Can you work these out from the model? Positions are in its coordinate system, mm. A direction names the side the tool comes from. Give positions to 0.01 mm unless a question says otherwise; leave off trailing zeros. Write each loop counter-clockwise with the first axis right and the second up, starting at its lowest first coordinate (ties: lowest second). Pieces come first, ordered by that corner, then holes. Notation, with made-up numbers: (8.25, 35) -> (63.25, 35) arc R20 cw to (63.25, 56) -> close; hole circle Ø1 at (70.5, 55.25). An arc over 180 degrees is marked (long way). One line per item, written item: value.
from build123d import *

# Parameters (mm, degrees)
SKETCH1_W             = 7.497163216
SKETCH1_H             = 13.3
SKETCH1_R             = 1
BOSS_EXTRUDE1_DEPTH   = 2
BOSS_EXTRUDE1_2_DEPTH = 2
SKETCH3_R             = 2.5
CUT_EXTRUDE1_DEPTH    = 1
BOSS_EXTRUDE3_DEPTH   = 1
SKETCH5_R             = 3.1
BOSS_EXTRUDE4_DEPTH   = 15.323280282
CUT_EXTRUDE2_REACH    = 37.51
SKETCH6_W             = 9.3
SKETCH6_H             = 13.397572085
BOSS_EXTRUDE5_START   = -13.397572085
BOSS_EXTRUDE5_DEPTH   = 13.397572085
SKETCH8_W             = 13.005673568
SKETCH8_H             = 3
BOSS_EXTRUDE6_DEPTH   = 10.5515
SKETCH9_W             = 13.3
SKETCH9_H             = 12.323280282
BOSS_EXTRUDE7_DEPTH   = 4
SKETCH10_W            = 4
SKETCH10_H            = 13.3
BOSS_EXTRUDE8_DEPTH   = 70
BOSS_EXTRUDE9_DEPTH   = 13.3
SKETCH15_W            = 4
SKETCH15_H            = 20
BOSS_EXTRUDE13_DEPTH  = 20
SKETCH16_W            = 4
SKETCH16_H            = 20
BOSS_EXTRUDE14_DEPTH  = 30
CUT_EXTRUDE3_DEPTH    = 20
BOSS_EXTRUDE15_DEPTH  = 4
BOSS_EXTRUDE16_DEPTH  = 20
SKETCH21_W            = 7.497163216
SKETCH21_H            = 9.3
CUT_EXTRUDE4_DEPTH    = 2
BOSS_EXTRUDE18_DEPTH  = 4
CUT_EXTRUDE5_DEPTH    = 4
BOSS_EXTRUDE20_DEPTH  = 8.1
FILLET1_R             = 5


with BuildPart() as part:
    # Sketch1 → Boss-Extrude1 (new body)
    with BuildSketch(Plane(origin=(0, 0, 0), x_dir=(1, 0, 0), z_dir=(0, 1, 0))):
        with Locations((6.360378056, -6.65)):
            Rectangle(SKETCH1_W, SKETCH1_H)
        with Locations(Location((6.360378056, -6.65, 0), (0, 0, 270))):
            Circle(SKETCH1_R, mode=Mode.SUBTRACT)
    extrude(amount=BOSS_EXTRUDE1_DEPTH)


with BuildPart() as body_2:
    # Sketch1 → Boss-Extrude1 2 (new body)
    with BuildSketch(Plane(origin=(0, 0, 0), x_dir=(1, 0, 0), z_dir=(0, 1, 0))):
        with Locations((26.86321484, -6.65)):
            Rectangle(SKETCH1_W, SKETCH1_H)
        with Locations(Location((26.86321484, -6.65, 0), (0, 0, 270))):
            Circle(SKETCH1_R, mode=Mode.SUBTRACT)
    extrude(amount=BOSS_EXTRUDE1_2_DEPTH)


with BuildPart() as cut_extrude1_tool:
    # Sketch3 → Cut-Extrude1 (new body)
    with BuildSketch(Plane(origin=(0, 2, 0), x_dir=(1, 0, 0), z_dir=(0, 1, 0))):
        with Locations(Location((26.86321484, -6.65, 0), (0, 0, 270))):
            Circle(SKETCH3_R)
        with Locations(Location((6.360378056, -6.65, 0), (0, 0, 270))):
            Circle(SKETCH3_R)
    extrude(amount=-CUT_EXTRUDE1_DEPTH)


with BuildPart() as part_1:
    add(part.part)

    # Cut-Extrude1: cut by cut_extrude1_tool
    add(cut_extrude1_tool.part, mode=Mode.SUBTRACT)



with BuildPart() as body_2_1:
    add(body_2.part)

    # Cut-Extrude1: cut by cut_extrude1_tool
    add(cut_extrude1_tool.part, mode=Mode.SUBTRACT)


with BuildPart() as part_2:
    add(part_1.part)

    add(body_2_1.part)  # Boss-Extrude3 merges body 2
    # Sketch4 → Boss-Extrude3 (add)
    with BuildSketch(Plane.XY.offset(13.3)):
        Polygon((10.108959664, 0), (10.108959664, -6.625791341), (23.114633232, -6.625791341), (23.114633232, 2), (10.108959664, 2), align=None)
    extrude(amount=-BOSS_EXTRUDE3_DEPTH)

    # Sketch5 → Boss-Extrude4 (add)
    with BuildSketch(Plane(origin=(0, 2, 0), x_dir=(1, 0, 0), z_dir=(0, 1, 0))):
        Polygon((10.108959664, 0), (2.611796448, 0), (2.611796448, -4), (2.611796448, -9.3), (2.611796448, -12.3), (2.611796448, -13.3), (30.611796448, -13.3), (30.611796448, -12.3), (30.611796448, -9.3), (30.611796448, -4), (30.611796448, 0), (23.114633232, 0), (23.114633232, -4), (23.114633232, -9.3), (23.114633232, -12.3), (10.108959664, -12.3), (10.108959664, -9.3), (10.108959664, -4), align=None)
        with Locations(Location((6.360378056, -6.65, 0), (0, 0, 270))):
            Circle(SKETCH5_R, mode=Mode.SUBTRACT)
        with Locations(Location((26.86321484, -6.65, 0), (0, 0, 270))):
            Circle(SKETCH5_R, mode=Mode.SUBTRACT)
    extrude(amount=BOSS_EXTRUDE4_DEPTH)

    # Cut-Extrude2: up to this face of the body (flat: up to its plane)
    cut_extrude2_end = Plane(part_2.part.faces().sort_by_distance((23.114633232, 8.661640141, 6.15))[0])
    # Sketch6 → Cut-Extrude2 (cut, up to the picked face)
    with BuildSketch(Plane(origin=(30.611796448, 0, 0), x_dir=(0, 0, -1), z_dir=(1, 0, 0)), mode=Mode.PRIVATE) as cut_extrude2_sk1:
        with Locations((-4.65, 10.62449424)):
            Rectangle(SKETCH6_W, SKETCH6_H)
    cut_extrude2_tool1 = split(extrude(cut_extrude2_sk1.sketch, amount=-CUT_EXTRUDE2_REACH, mode=Mode.PRIVATE), bisect_by=cut_extrude2_end, keep=Keep.BOTH, mode=Mode.PRIVATE)
    add(cut_extrude2_tool1.solids().sort_by(Axis((30.611796, 10.624494, 4.65), (-1, 0, 0)))[0], mode=Mode.SUBTRACT)

    # Sketch7 → Boss-Extrude5 (add)
    with BuildSketch(Plane(origin=(0, 17.323280282, 0), x_dir=(1, 0, 0), z_dir=(0, 1, 0)).offset(BOSS_EXTRUDE5_START)):
        with BuildLine():
            Line((28.471785634, -9.3), (30.611796448, -9.3))
            Line((30.611796448, -9.3), (30.611796448, -13.3))
            Line((30.611796448, -13.3), (10.108959664, -13.3))
            Line((10.108959664, -13.3), (10.108959664, -9.3))
            Line((10.108959664, -9.3), (25.254644046, -9.3))
            ThreePointArc((25.254644046, -9.3), (26.86321484, -9.75), (28.471785634, -9.3))
        make_face()
    extrude(amount=BOSS_EXTRUDE5_DEPTH)

    # Sketch8 → Boss-Extrude6 (add, through all)
    with BuildSketch(Plane.XZ.offset(-3.925708197)):
        with Locations((16.611796448, 10.8)):
            Rectangle(SKETCH8_W, SKETCH8_H)
    extrude(amount=BOSS_EXTRUDE6_DEPTH)

    # Sketch9 → Boss-Extrude7 (add)
    with BuildSketch(Plane.ZY.offset(-2.611796448)):
        with Locations((6.65, 11.161640141)):
            Rectangle(SKETCH9_W, SKETCH9_H)
    extrude(amount=BOSS_EXTRUDE7_DEPTH)

    # Sketch10 → Boss-Extrude8 (add)
    with BuildSketch(Plane(origin=(0, 17.323280282, 0), x_dir=(1, 0, 0), z_dir=(0, 1, 0))):
        with Locations((0.611796448, -6.65)):
            Rectangle(SKETCH10_W, SKETCH10_H)
    extrude(amount=BOSS_EXTRUDE8_DEPTH)

    # Sketch11 → Boss-Extrude9 (add)
    with BuildSketch(Plane.XY.offset(13.3)):
        Polygon((-1.388203552, 5), (2.611796448, 0), (2.611796448, 5), align=None)
    extrude(amount=-BOSS_EXTRUDE9_DEPTH)

    # Sketch15 → Boss-Extrude13 (add)
    with BuildSketch(Plane.XY.offset(13.3)):
        with Locations((0.611796448, 47.323280282)):
            Rectangle(SKETCH15_W, SKETCH15_H)
    extrude(amount=BOSS_EXTRUDE13_DEPTH)

    # Sketch16 → Boss-Extrude14 (add)
    with BuildSketch(Plane(origin=(0, 57.323280282, 0), x_dir=(1, 0, 0), z_dir=(0, 1, 0))):
        with Locations((0.611796448, -23.3)):
            Rectangle(SKETCH16_W, SKETCH16_H)
    extrude(amount=BOSS_EXTRUDE14_DEPTH)

    # Sketch17 → Cut-Extrude3 (cut)
    with BuildSketch(Plane.ZY.offset(1.388203552)):
        Polygon((13.3, 87.323280282), (0, 87.323280282), (0, 57.323280282), (0, 44.023280282), (13.3, 57.323280282), align=None)
        Polygon((33.3, 87.323280282), (26.6, 87.323280282), (26.6, 50.623280282), (13.3, 37.323280282), (26.6, 37.323280282), (33.3, 37.323280282), align=None)
    extrude(amount=-CUT_EXTRUDE3_DEPTH, mode=Mode.SUBTRACT)

    # Sketch18 → Boss-Extrude15 (add)
    with BuildSketch(Plane.ZY.offset(1.388203552)):
        Polygon((3.495517328, 77.823280282), (36.404482672, 96.823280282), (36.404482672, 92.823280282), (3.495517328, 73.823280282), align=None)
        Polygon((3.495517328, 56.502772207), (36.404482672, 75.502772207), (36.404482672, 71.502772207), (3.495517328, 52.502772207), align=None)
    extrude(amount=-BOSS_EXTRUDE15_DEPTH)

    # Sketch19 → Boss-Extrude16 (add)
    with BuildSketch(Plane.ZY.offset(1.388203552)):
        Polygon((3.495517328, 77.823280282), (6.959618943, 79.823280282), (6.959618943, 75.823280282), (3.495517328, 73.823280282), align=None)
        Polygon((3.495517328, 56.502772207), (6.959618943, 58.502772207), (6.959618943, 54.502772207), (3.495517328, 52.502772207), align=None)
        Polygon((36.404482672, 75.502772207), (32.940381057, 73.502772207), (32.940381057, 69.502772207), (36.404482672, 71.502772207), align=None)
        Polygon((36.404482672, 92.823280282), (32.940381057, 90.823280282), (32.940381057, 94.823280282), (36.404482672, 96.823280282), align=None)
    extrude(amount=BOSS_EXTRUDE16_DEPTH)

    # Sketch21 → Cut-Extrude4 (cut)
    with BuildSketch(Plane(origin=(0, 3.925708197, 0), x_dir=(1, 0, 0), z_dir=(0, 1, 0))):
        with Locations((26.86321484, -4.65)):
            Rectangle(SKETCH21_W, SKETCH21_H)
    extrude(amount=-CUT_EXTRUDE4_DEPTH, mode=Mode.SUBTRACT)

    # Sketch22 → Boss-Extrude18 (add)
    with BuildSketch(Plane.ZY.offset(21.388203552)):
        Polygon((3.495517328, 77.823280282), (36.404482672, 96.823280282), (36.404482672, 92.823280282), (3.495517328, 73.823280282), align=None)
        Polygon((3.495517328, 56.502772207), (3.495517328, 52.502772207), (36.404482672, 71.502772207), (36.404482672, 75.502772207), align=None)
    extrude(amount=BOSS_EXTRUDE18_DEPTH)

    # Sketch23 → Cut-Extrude5 (cut)
    with BuildSketch(Plane(origin=(2.611796448, 0, 0), x_dir=(0, 0, -1), z_dir=(1, 0, 0))):
        Polygon((-13.3, 87.323280282), (-13.3, 83.483900992), (-19.95, 87.323280282), align=None)
    extrude(amount=-CUT_EXTRUDE5_DEPTH, mode=Mode.SUBTRACT)

    # Sketch24 → Boss-Extrude20 (add)
    with BuildSketch(Plane(origin=(2.611796448, 0, 0), x_dir=(0, 0, -1), z_dir=(1, 0, 0))):
        Polygon((-26.6, 91.162659572), (-13.300321898, 83.48408684), (-13.3, 62.163392916), (-26.599678102, 69.841965649), align=None)
    extrude(amount=BOSS_EXTRUDE20_DEPTH)

    # Fillet1
    # the kernel refuses this fillet: 5 mm, written as the material it takes off along each edge
    with BuildSketch(Plane(origin=(30.611796448, 17.323280282, -3.2), x_dir=(-1, 0, 0), z_dir=(0, 0, 1))) as fillet1_piece_1:
        with BuildLine():
            CenterArc((FILLET1_R, FILLET1_R), FILLET1_R, 180, 90)
            Line((0, FILLET1_R), (0, 0))
            Line((0, 0), (FILLET1_R, 0))
        make_face()
    extrude(amount=29, mode=Mode.SUBTRACT)


solid = part_2.part
1) We'd pull the mould along Z, two halves only. Please class faces 1 (the face through (27, 1, 8)), 2 (the face through (6.61, 65.95, 19.86)), 3 (the face through (-12, 54, 3.496)), 4 (the face through (3.334, 9.554, 5.978)): released by +Z, released by -Z, zero draft, split by the parting line, or undercut.
Answer list:
face 1: undercut
face 2: released by +Z
face 3: released by -Z
face 4: undercut
2) If we section it at A-A (x = -14): Write out the boundary of the cut face in (y, z), and give its area (3 significant figures).
Answer list:
outline: (52.5, 3.5) -> (56.5, 3.5) -> (58.5, 6.96) -> (54.5, 6.96) -> close; (69.5, 32.94) -> (73.5, 32.94) -> (75.5, 36.4) -> (71.5, 36.4) -> close; (73.82, 3.5) -> (77.82, 3.5) -> (79.82, 6.96) -> (75.82, 6.96) -> close; (90.82, 32.94) -> (94.82, 32.94) -> (96.82, 36.4) -> (92.82, 36.4) -> close
area: 55.4 mm^2
3) Will these pins go through, and if not, where does the flat tip stop? pin 1 (12 mm diameter, centred on x = 2.5, y = 33.5, fed in from +Z); pin 2 (1.2 mm diameter, centred on x = 0.5, y = 61, fed in from +Z); pin 3 (5.5 mm diameter, centred on y = 62.5, z = 20.5, fed in from +X).
Answer list:
pin 1: stops at z = 15.48
pin 2: stops at z = 26.6
pin 3: stops at x = 2.61
4) I need wall thicknesses on L1, parallel to X at y = 32.5, z = 11.5; L2, parallel to X at y = 0.65, z = 6.65; L3, parallel to X at y = 64, z = 19.5. Which ranges of each line are inside material? Lowest first, please.
Answer list:
L1: x = -1.39 to 2.61
L2: x = 2.09 to 5.36, 7.36 to 10.11, 23.11 to 25.86, 27.86 to 30.61
L3: x = -25.39 to -21.39, -1.39 to 2.61
5) If we section it at C-C (x = 22): Write out the boundary of the cut face in (y, z), and give its area (3 significant figures).
Answer list:
outline: (-6.63, 9.3) -> (17.32, 9.3) -> (17.32, 13.3) -> (-6.63, 13.3) -> close
area: 95.8 mm^2
6) For faces 5 (the face through (2.612, 78, 8)), 6 (the face through (-21.388, 63, 20)), 7 (the face through (6, 0, 8)), which set-ups out of +Z, -Z, +X, -X, +Y, -Y let a thin tool reach every point of the face, with its end or its side?
Answer list:
face 5: -Z, +X, +Y
face 6: +Y, -Y
face 7: +Z, -Z, -X, -Y
7) If we section it at B-B (z = 24.5): Write out the boundary of the cut face in (x, y), and give its area (3 significant figures).
Answer list:
outline: (-25.39, 64.63) -> (-21.39, 64.63) -> (-21.39, 68.63) -> (-25.39, 68.63) -> close; (-25.39, 85.95) -> (-21.39, 85.95) -> (-21.39, 89.95) -> (-25.39, 89.95) -> close; (-1.39, 48.52) -> (2.61, 48.52) -> (2.61, 68.63) -> (10.71, 68.63) -> (10.71, 89.95) -> (-1.39, 89.95) -> close
area: 370 mm^2
